from build123d import *

# Parameters (mm, degrees)
PAD001_DEPTH    = 18
POCKET001_DEPTH = 18
SKETCH004_W     = 19
SKETCH004_H     = 420
POCKET002_DEPTH = 9.5
POCKET004_DEPTH = 12


with BuildPart() as part:
    # Sketch002 → Pad001 (new body)
    with BuildSketch(Plane.XY):
        with BuildLine():
            Line((-360, 420), (360, 420))
            Line((360, 420), (360, 36))
            ThreePointArc((324, 0), (349.455844, 10.544156), (360, 36))
            Line((324, 0), (-324, 0))
            ThreePointArc((-360, 36), (-349.455844, 10.544156), (-324, 0))
            Line((-360, 36), (-360, 420))
        make_face()
    extrude(amount=PAD001_DEPTH)

    # Sketch003 → Pocket001 (cut)
    with BuildSketch(Plane.XY.offset(18)):
        with BuildLine():
            ThreePointArc((-274, 253), (-290, 269), (-306, 253))
            Line((-306, 253), (-306, 73))
            ThreePointArc((-306, 73), (-290, 57), (-274, 73))
            Line((-274, 73), (-274, 253))
        make_face()
        with BuildLine():
            ThreePointArc((-136.333333, 253), (-152.333333, 269), (-168.333333, 253))
            Line((-168.333333, 253), (-168.333333, 73))
            ThreePointArc((-168.333333, 73), (-152.333333, 57), (-136.333333, 73))
            Line((-136.333333, 73), (-136.333333, 253))
        make_face()
        with BuildLine():
            ThreePointArc((306, 253), (290, 269), (274, 253))
            Line((274, 73), (274, 253))
            ThreePointArc((274, 73), (290, 57), (306, 73))
            Line((306, 253), (306, 73))
        make_face()
        with BuildLine():
            ThreePointArc((168.333333, 253), (152.333333, 269), (136.333333, 253))
            Line((136.333333, 73), (136.333333, 253))
            ThreePointArc((136.333333, 73), (152.333333, 57), (168.333333, 73))
            Line((168.333333, 253), (168.333333, 73))
        make_face()
        with BuildLine():
            Line((-27, 324), (27, 324))
            ThreePointArc((39, 312), (35.485281, 320.485281), (27, 324))
            Line((39, 312), (39, 148))
            ThreePointArc((27, 136), (35.485281, 139.514719), (39, 148))
            Line((27, 136), (-27, 136))
            ThreePointArc((-39, 148), (-35.485281, 139.514719), (-27, 136))
            Line((-39, 148), (-39, 312))
            ThreePointArc((-27, 324), (-35.485281, 320.485281), (-39, 312))
        make_face()
    extrude(amount=-POCKET001_DEPTH, mode=Mode.SUBTRACT)

    # Sketch004 → Pocket002 (cut)
    with BuildSketch(Plane.XY.offset(18)):
        with Locations((-100, 210)):
            Rectangle(SKETCH004_W, SKETCH004_H)
        with Locations((100, 210)):
            Rectangle(SKETCH004_W, SKETCH004_H)
    extrude(amount=-POCKET002_DEPTH, mode=Mode.SUBTRACT)

    # Sketch007 → Pocket004 (cut)
    with BuildSketch(Plane.XY.offset(18)):
        with BuildLine():
            Line((-27, 330), (27, 330))
            ThreePointArc((45, 312), (39.727922, 324.727922), (27, 330))
            Line((45, 312), (45, 148))
            ThreePointArc((27, 130), (39.727922, 135.272078), (45, 148))
            Line((27, 130), (-27, 130))
            ThreePointArc((-45, 148), (-39.727922, 135.272078), (-27, 130))
            Line((-45, 148), (-45, 312))
            ThreePointArc((-27, 330), (-39.727922, 324.727922), (-45, 312))
        make_face()
    extrude(amount=-POCKET004_DEPTH, mode=Mode.SUBTRACT)


with BuildPart() as part_1:
    # Body001 placement: moved
    add(part.part.moved(Location((0, 0, 18))))


solid = part_1.part
The model under review builds one solid part; all positions refer to its coordinate system, in mm. A direction names the side the tool comes from. Give positions to 0.01 mm unless a question says otherwise; leave off trailing zeros. Loops run counter-clockwise (first coordinate to the right, second up) from the corner with the lowest first, then second, coordinate; pieces in that order, holes last. Notation, with made-up numbers: (-33.75, -31) -> (-12.75, -31) arc R29 ccw to (-12.75, -4) -> close; hole circle Ø7 at (67, 12). An arc over 180 degrees is marked (long way). Put each result on its own line as item: value. Start each with the question number.
1. We need section A-A on x = 290. State the section outline as (y, z) points.
2. Clearance check with a flat-ended pin moving along its axis: P1, Ø9.5, axis at x = 102.5, y = 222, coming from the +Z side. State where the tip first meets the part, or that it passes through.
3. We need section C-C on x = 151. State the section outline as (y, z) points.
4. We need section B-B on y = 338. State the section outline as (x, z) points.
5. Mouldability with a two-part tool opening along X and no side actions: class faces 4 (the face through (-39.587, 324.867, 30.084)), 5 (the face through (-360, 225, 27)), 6 (the face through (40, 238, 24)), 7 (the face through (62, 213, 36)) as released by +X, released by -X, zero draft, split by the parting line, or undercut.
6. For faces 1 (the face through (5, 0, 27)), 2 (the face through (151.982, 57.004, 27.126)), 3 (the face through (-100, 213, 26.5)), list the 3-axis set-ups (+Z, -Z, +X, -X, +Y, -Y) from which the entire face can be reached by the end or side of a thin tool; tool diameter is ignored.
7. We need section D-D on y = 159. State how many separate pieces and enclosed holes the cut face has, then the cut area to 3 significant figures.
8. Wall thickness on probe 1 along X at (y, z) = (252, 25.5); probe 2 along X at (y, z) = (297.5, 32); probe 3 along X at (y, z) = (91, 21): over which ranges is each line inside the solid? List them lowest first.
Determined:
1. outline: (0, 18) -> (57, 18) -> (57, 36) -> (0, 36) -> close; (269, 18) -> (420, 18) -> (420, 36) -> (269, 36) -> close
2. P1: z = 26.5
3. outline: (0, 18) -> (57.06, 18) -> (57.06, 36) -> (0, 36) -> close; (268.94, 18) -> (420, 18) -> (420, 36) -> (268.94, 36) -> close
4. outline: (-360, 18) -> (360, 18) -> (360, 36) -> (109.5, 36) -> (109.5, 26.5) -> (90.5, 26.5) -> (90.5, 36) -> (-90.5, 36) -> (-90.5, 26.5) -> (-109.5, 26.5) -> (-109.5, 36) -> (-360, 36) -> close
5. face 4: undercut
5. face 5: released by -X
5. face 6: undercut
5. face 7: zero draft
6. face 1: +Z, -Z, +X, -X, -Y
6. face 2: +Z, -Z
6. face 3: +Z, +Y, -Y
7. separate pieces: 6
7. enclosed holes: 0
7. area: 8,750 mm^2
8. probe 1: -360 to -306, -274 to -168.33, -136.33 to -45, 45 to 136.33, 168.33 to 274, 306 to 360
8. probe 2: -360 to -109.5, -90.5 to -45, 45 to 90.5, 109.5 to 360
8. probe 3: -360 to -306, -274 to -168.33, -136.33 to 136.33, 168.33 to 274, 306 to 360
